from build123d import *

# Parameters (mm, degrees)
SKETCH1_R             = 0.5
FRONT_FACE_EXT_DEPTH  = 1
SKETCH2_W             = 1
SKETCH2_H             = 6.5
LENGTH_EXTRUDE1_DEPTH = 1.7874
SKETCH3_W             = 1
SKETCH3_H             = 1
BOSS_EXTRUDE2_DEPTH   = 1
SKETCH4_W             = 9.4574
SKETCH4_H             = 1
HEIGHT_EXTRUDE3_DEPTH = 2.5874
SKETCH5_W             = 1
SKETCH5_H             = 1
BOSS_EXTRUDE4_DEPTH   = 1
SKETCH6_W             = 7.33
SKETCH6_H             = 1
BOSS_EXTRUDE5_DEPTH   = 0.8


with BuildPart() as part:
    # Sketch1 → Front Face Ext (new body)
    with BuildSketch(Plane.XY):
        with BuildLine():
            Line((-0.75, -3.25), (-7.5, -3.25))
            Line((-7.5, -3.25), (-7.5, 3.25))
            Line((-7.5, 3.25), (7.5, 3.25))
            Line((7.5, 3.25), (7.5, -3.25))
            Line((7.5, -3.25), (0.25, -3.25))
            ThreePointArc((0.25, -3.25), (-0.25, -2.75), (-0.75, -3.25))
        make_face()
        with Locations((-5.5, 2.25)):
            Circle(SKETCH1_R, mode=Mode.SUBTRACT)
        with Locations((6.5, -0.25)):
            Circle(SKETCH1_R, mode=Mode.SUBTRACT)
    extrude(amount=FRONT_FACE_EXT_DEPTH)

    # Sketch2 → Length-Extrude1 (add)
    with BuildSketch(Plane.ZY.offset(7.5)):
        with Locations((0.5, 0)):
            Rectangle(SKETCH2_W, SKETCH2_H)
    extrude(amount=LENGTH_EXTRUDE1_DEPTH)

    # Sketch3 → Boss-Extrude2 (add)
    with BuildSketch(Plane.XY.offset(1)):
        with Locations((-8.7874, 2.75)):
            Rectangle(SKETCH3_W, SKETCH3_H)
        with Locations((-8.7874, -2.75)):
            Rectangle(SKETCH3_W, SKETCH3_H)
    extrude(amount=BOSS_EXTRUDE2_DEPTH)

    # Sketch4 → Height-Extrude3 (add)
    with BuildSketch(Plane(origin=(0, 3.25, 0), x_dir=(1, 0, 0), z_dir=(0, 1, 0))):
        with Locations((-4.5587, -0.5)):
            Rectangle(SKETCH4_W, SKETCH4_H)
    extrude(amount=HEIGHT_EXTRUDE3_DEPTH)

    # Sketch5 → Boss-Extrude4 (add)
    with BuildSketch(Plane.XY.offset(1)):
        with Locations((-0.33, 5.3374)):
            Rectangle(SKETCH5_W, SKETCH5_H)
        with Locations((-3.94, 5.3374)):
            Rectangle(SKETCH5_W, SKETCH5_H)
    extrude(amount=BOSS_EXTRUDE4_DEPTH)

    # Sketch6 → Boss-Extrude5 (add)
    with BuildSketch(Plane(origin=(0, 3.25, 0), x_dir=(1, 0, 0), z_dir=(0, 1, 0))):
        with Locations((3.835, -0.5)):
            Rectangle(SKETCH6_W, SKETCH6_H)
    extrude(amount=BOSS_EXTRUDE5_DEPTH)


solid = part.part
Here's how the part is built. I have some questions about the finished solid (model axes, mm). A direction names the side the tool comes from. Give positions to 0.01 mm unless a question says otherwise; leave off trailing zeros. Order: outer loops, then holes, each group sorted by start corner. A loop starts at its lowest first (then second) coordinate and runs counter-clockwise, first axis right, second up. Notation, with made-up numbers: (-7.75, -34) -> (6.25, -34) arc R12 cw to (6.25, -19) -> close; hole circle Ø2 at (56, 49.25). An arc over 180 degrees is marked (long way). One line per item, written item: value. Start each with the question number.
1. Imagine slicing it at A-A, the plane x = 6.5. List the corners of the cut face in (y, z) for me, plus the area to 3 significant figures.
2. Imagine slicing it at C-C, the plane y = 5.5. List the corners of the cut face in (x, z) for me, plus the area to 3 significant figures.
3. For faces 4 (the face through (-8.287, 2.7, 1.5)), 5 (the face through (-3.44, 5.3, 1.5)), 6 (the face through (0.17, 5, 1)), 7 (the face through (-4.44, 5.3, 1.5)), which set-ups out of +Z, -Z, +X, -X, +Y, -Y let a thin tool reach every point of the face, with its end or its side?
4. We'd pull the mould along Y, two halves only. Please class faces 1 (the face through (-1, 1, 0)), 2 (the face through (-8.8, -2.25, 1.5)), 3 (the face through (-8.8, 3.25, 1.5)): released by +Y, released by -Y, zero draft, split by the parting line, or undercut.
5. Imagine slicing it at B-B, the plane z = 0.65. List the corners of the cut face in (x, y) for me.
6. Will these pins go through, and if not, where does the flat tip stop? pin 1 Ø0.8 at (x, z) = (-0.5, 1.5) entering from -Y; pin 2 Ø1.1 at (x, z) = (3.5, 0.5) entering from +Y; pin 3 Ø0.8 at (y, z) = (5, 1.5) entering from +X.
7. I need wall thicknesses on probe 1 along Y at (x, z) = (-5.5, 0.75); probe 2 along Y at (x, z) = (6.5, 0.55); probe 3 along X at (y, z) = (3, 1.6). Which ranges of each line are inside material? Lowest first, please. Write a range as from..to.
8. Imagine slicing it at D-D, the plane z = 1.35. List the corners of the cut face in (x, y) for me.
Values follow:
1. outline: (-3.25, 0) -> (-0.75, 0) -> (-0.75, 1) -> (-3.25, 1) -> close; (0.25, 0) -> (4.05, 0) -> (4.05, 1) -> (0.25, 1) -> close
1. area: 6.30 mm2
2. outline: (-9.29, 0) -> (0.17, 0) -> (0.17, 2) -> (-0.83, 2) -> (-0.83, 1) -> (-3.44, 1) -> (-3.44, 2) -> (-4.44, 2) -> (-4.44, 1) -> (-9.29, 1) -> close
2. area: 11.5 mm2
3. face 4: +Z, +X, +Y, -Y
3. face 5: +Z, +Y, -Y
3. face 6: +Z, -Z, +X, +Y
3. face 7: +Z, -X, +Y, -Y
4. face 1: zero draft
4. face 2: undercut
4. face 3: released by +Y
5. outline: (-9.29, -3.25) -> (-0.75, -3.25) arc R0.5 cw to (0.25, -3.25) -> (7.5, -3.25) -> (7.5, 4.05) -> (0.17, 4.05) -> (0.17, 5.84) -> (-9.29, 5.84) -> close; hole circle Ø1 at (-5.5, 2.25); hole circle Ø1 at (6.5, -0.25)
6. pin 1: stops at y = 4.84
6. pin 2: stops at y = 4.05
6. pin 3: stops at x = 0.17
7. probe 1: y = -3.25..1.75, 2.75..5.84
7. probe 2: y = -3.25..-0.75, 0.25..4.05
7. probe 3: x = -9.29..-8.29
8. outline: (-9.29, -3.25) -> (-8.29, -3.25) -> (-8.29, -2.25) -> (-9.29, -2.25) -> close; (-9.29, 2.25) -> (-8.29, 2.25) -> (-8.29, 3.25) -> (-9.29, 3.25) -> close; (-4.44, 4.84) -> (-3.44, 4.84) -> (-3.44, 5.84) -> (-4.44, 5.84) -> close; (-0.83, 4.84) -> (0.17, 4.84) -> (0.17, 5.84) -> (-0.83, 5.84) -> close
